Input: part model. Units: mm. Frame: model coordinates. A direction names the side the tool comes from. Give positions to 0.01 mm unless a question says otherwise; leave off trailing zeros. Loops run counter-clockwise (first coordinate to the right, second up) from the corner with the lowest first, then second, coordinate; pieces in that order, holes last. Notation, with made-up numbers: (-23.5, 49.25) - (-4.5, 49.25) arc R15 cw to (-4.5, 70.25) - close; hole circle Ø7 at (-16.5, -4). An arc over 180 degrees is marked (long way). Answer as a JSON object with one key per item and string values.
from build123d import *

# Parameters (mm, degrees)
F0_W     = 25.4
F0_H     = 25.4
F1_DEPTH = 50.8
F2_W     = 38.1
F2_H     = 31.75
F3_DEPTH = 50.801
F4_R     = 12.7
F5_R     = 12.7
F7_DEPTH = 76.2
F8_W     = 50.8
F8_H     = 25.4
F9_DEPTH = 136.3117039084


with BuildPart() as f1:
    # F0 (on Front) → F1 (new body, symmetric)
    with BuildSketch(Plane.XZ):
        with Locations((-10.1491656572, 12.7)):
            Rectangle(F0_W, F0_H)
        with Locations((91.4508343428, 12.7)):
            Rectangle(F0_W, F0_H)
        Polygon((-22.8491656572, 25.4), (2.5508343428, 25.4), (78.7508343428, 25.4), (104.1508343428, 25.4), (127, 25.4), (142.2508343428, 25.4), (142.2508343428, 50.8), (-60.9491656572, 50.8), (-60.9491656572, 25.4), align=None)
    extrude(amount=F1_DEPTH, both=True)

    # F2 (on face) → F3 (cut, through all)
    with BuildSketch(Plane.XY.offset(50.8)):
        with Locations((-41.8991656572, 3.175)):
            Rectangle(F2_W, F2_H)
        with Locations((123.2008343428, 3.175)):
            Rectangle(F2_W, F2_H)
    extrude(amount=-F3_DEPTH, mode=Mode.SUBTRACT)

    # F4
    f4_edges = [f1.edges().sort_by_distance(p)[0] for p in [
        (142.250834, -50.8, 38.1),
        (142.250834, 50.8, 38.1),
        (-60.949166, -50.8, 38.1),
        (-60.949166, 50.8, 38.1),
    ]]
    fillet(f4_edges, radius=F4_R)

    # F5
    f5_edges = [f1.edges().sort_by_distance(p)[0] for p in [
        (2.550834, 0, 25.4),
        (78.750834, 0, 25.4),
    ]]
    fillet(f5_edges, radius=F5_R)

    # F6 (on face) → F7 (join)
    with BuildSketch(Plane.XY.offset(50.8)):
        Polygon((91.4508343428, 50.8), (40.6508343428, 50.8), (-10.1491656572, 50.8), (40.6508343428, -50.8), align=None)
    extrude(amount=F7_DEPTH)

    # F8 (on face) → F9 (cut, through all)
    with BuildSketch(Plane(origin=(52.8406674742, -26.4203337371, 0), x_dir=(0.4472135955, 0.894427191, 0), z_dir=(0.894427191, -0.4472135955, 0))):
        with Locations((-1.8572955163, 88.9)):
            Rectangle(F8_W, F8_H)
    extrude(amount=-F9_DEPTH, mode=Mode.SUBTRACT)


solid = f1.part
Item 1: Cut plane A-A (x = -46). Return loops of the section in (y, z), then the cut area to 3 significant figures.
Geometry check:
{"outline": "(-50.8, 25.4) - (-12.7, 25.4) - (-12.7, 50.8) - (-50.8, 50.8) - close; (19.05, 25.4) - (50.8, 25.4) - (50.8, 50.8) - (19.05, 50.8) - close", "area": "1,770 mm2"}
Item 2: Material intervals for line 1 (Z direction, x = -18, y = 24); line 2 (X direction, y = 14.5, z = 33); line 3 (Z direction, x = 52.5, y = 35.5), sorted ascending. Write a range as [from, to].
Geometry check:
{"line 1": "z = [0, 50.8]", "line 2": "x = [-22.85, 104.15]", "line 3": "z = [25.4, 127]"}
Item 3: Access query for faces 1 (the face through (123, 19.05, 38)), 2 (the face through (2.551, -1, 6)), 3 (the face through (123, 35, 25.4)), 4 (the face through (40, -10, 101.6)), 5 (the face through (-42, -12.7, 38)). Directions: +Z, -Z, +X, -X, +Y, -Y. A direction counts if a zero-diameter tool reaches every point of the face in a straight line with its end or side. Return the directions, or none.
Geometry check:
{"face 1": "+Z, -Z, +X", "face 2": "-Z, +Y, -Y", "face 3": "-Z, +X, +Y, -Y", "face 4": "-X, -Y", "face 5": "+Z, -Z, -X"}
Item 4: Contact query for flat-ended pins moving along their axis: P1, Ø11.5, axis at x = -50.5, y = -33, coming from the -Z side; P2, Ø4, axis at x = 13, z = 90, coming from the -Y side; P3, Ø10, axis at x = -24.5, z = 13, coming from the +Y side; P4, Ø10, axis at y = -6, z = 7, coming from the +X side. Output: stop coordinate, or through.
Geometry check:
{"P1": "stops at z = 25.4", "P2": "stops at y = 18.82", "P3": "stops at y = 50.8", "P4": "stops at x = 104.15"}
Item 5: Mould query, pull axis X, two halves, no side actions, for faces 6 (the face through (78.751, -1, 6)), 7 (the face through (-60.949, -26, 38)), 8 (the face through (91, -1, 0)). Classes: released by +X, released by -X, zero draft, split by the parting line, or undercut.
Geometry check:
{"face 6": "undercut", "face 7": "released by -X", "face 8": "zero draft"}
Item 6: Cut plane C-C (z = 31.5). Return loops of the section in (x, y).
Geometry check:
{"outline": "(-60.95, -38.1) arc R12.7 ccw to (-48.25, -50.8) - (129.55, -50.8) arc R12.7 ccw to (142.25, -38.1) - (142.25, -12.7) - (104.15, -12.7) - (104.15, 19.05) - (142.25, 19.05) - (142.25, 38.1) arc R12.7 ccw to (129.55, 50.8) - (-48.25, 50.8) arc R12.7 ccw to (-60.95, 38.1) - (-60.95, 19.05) - (-22.85, 19.05) - (-22.85, -12.7) - (-60.95, -12.7) - close"}
Item 7: Cut plane D-D (y = 5.5). Return loops of the section in (x, z), then the cut area to 3 significant figures.
Geometry check:
{"outline": "(-22.85, 0) - (2.55, 0) - (2.55, 12.7) arc R12.7 cw to (15.25, 25.4) - (66.05, 25.4) arc R12.7 cw to (78.75, 12.7) - (78.75, 0) - (104.15, 0) - (104.15, 50.8) - (68.8, 50.8) - (68.8, 127) - (12.5, 127) - (12.5, 101.6) - (41.64, 101.6) - (41.64, 76.2) - (12.5, 76.2) - (12.5, 50.8) - (-22.85, 50.8) - close", "area": "8,140 mm2"}
Item 8: Cut plane B-B (y = -26). Return loops of the section in (x, z), then the cut area to 3 significant figures.
Geometry check:
{"outline": "(-60.95, 25.4) - (-22.85, 25.4) - (-22.85, 0) - (2.55, 0) - (2.55, 12.7) arc R12.7 cw to (15.25, 25.4) - (66.05, 25.4) arc R12.7 cw to (78.75, 12.7) - (78.75, 0) - (104.15, 0) - (104.15, 25.4) - (142.25, 25.4) - (142.25, 50.8) - (53.05, 50.8) - (53.05, 76.2) - (28.25, 76.2) - (28.25, 50.8) - (-60.95, 50.8) - close; (28.25, 101.6) - (53.05, 101.6) - (53.05, 127) - (28.25, 127) - close", "area": "7,780 mm2"}
